Geometry: final body of the model. Coordinates: model frame, mm. A direction names the side the tool comes from. Round coordinates to 2 decimals unless told otherwise and drop trailing zeros. Loops run counter-clockwise (first coordinate to the right, second up) from the corner with the lowest first, then second, coordinate; pieces in that order, holes last. Notation, with made-up numbers: (8, -27) - (27, -27) arc R9 cw to (27, -13) - close; hole circle Ø4 at (-11.5, -23). An arc over 180 degrees is marked (long way). Answer as CSV lines item,"result".
from build123d import *

# Parameters (mm, degrees)
BOSS_EXTRUDE1_DEPTH       = 76.2
TAP_DRILL_FOR_6_32_TAP1_D = 2.7051


with BuildPart() as part:
    # Sketch2 → Boss-Extrude1 (new body)
    with BuildSketch(Plane.XY):
        with BuildLine():
            Line((-19.425899611, -6.35), (-6.35, -6.35))
            Line((-6.35, -6.35), (-6.35, 0))
            ThreePointArc((-6.35, 0), (0, 6.35), (6.35, 0))
            Line((6.35, 0), (6.35, -6.35))
            Line((6.35, -6.35), (19.425899611, -6.35))
            Line((19.425899611, -6.35), (19.425899611, -3.175))
            Line((19.425899611, -3.175), (12.7, -3.175))
            Line((12.7, -3.175), (12.7, 0))
            ThreePointArc((12.7, 0), (0, 12.7), (-12.7, 0))
            Line((-12.7, 0), (-12.7, -3.175))
            Line((-12.7, -3.175), (-19.425899611, -3.175))
            Line((-19.425899611, -3.175), (-19.425899611, -6.35))
        make_face()
    extrude(amount=BOSS_EXTRUDE1_DEPTH)

    # Tap Drill for #6-32 Tap1 (through all)
    with Locations(Plane(origin=(0, -3.175, 0), x_dir=(1, 0, 0), z_dir=(0, 1, 0))):
        with Locations((-16.062949805, -38.1), (16.062949805, -38.1)):
            Hole(TAP_DRILL_FOR_6_32_TAP1_D / 2)


solid = part.part
(1) Pin query (flat end, axial travel): P1, Ø2.5, axis at x = 16.06, z = 38.1, coming from the -Y side; P2, Ø5, axis at x = -1.5, z = 25, coming from the -Y side; P3, Ø3, axis at y = -1, z = 21.5, coming from the -X side; P4, Ø5, axis at x = -9.5, z = 36.5, coming from the +Y side. Return the tip coordinate at first contact, or that it passes through.
Findings below:
P1,"through"
P2,"y = 4.93"
P3,"x = -12.7"
P4,"y = 10.6"
(2) Section B-B (z = 50.5). Output: boundary loops of the cut face in (x, y) (3 decimals).
Findings below:
outline,"(-19.426, -6.35) - (-6.35, -6.35) - (-6.35, 0) arc R6.35 cw to (6.35, 0) - (6.35, -6.35) - (19.426, -6.35) - (19.426, -3.175) - (12.7, -3.175) - (12.7, 0) arc R12.7 ccw to (-12.7, 0) - (-12.7, -3.175) - (-19.426, -3.175) - close"
(3) Section C-C (x = 0). Output: boundary loops of the cut face in (y, z).
Findings below:
outline,"(6.35, 0) - (12.7, 0) - (12.7, 76.2) - (6.35, 76.2) - close"
(4) Section D-D (y = 8.5). Output: boundary loops of the cut face in (x, z), and give its area (3 significant figures).
Findings below:
outline,"(-9.44, 0) - (9.44, 0) - (9.44, 76.2) - (-9.44, 76.2) - close"
area,"1,440 mm2"
(5) Draft query along X for faces 1 (the face through (15.44, -4.78, 39.3)), 2 (the face through (0.279, 12.697, 37.567)), 3 (the face through (-6.35, -3, 38)), 4 (the face through (-19.426, -5, 38)). Return one class per face: pulls with the +X half, pulls with the -X half, needs draft (parallel to the pull), parting line crosses it, or undercut.
Findings below:
face 1,"undercut"
face 2,"parting line crosses it"
face 3,"undercut"
face 4,"pulls with the -X half"
(6) Section A-A (x = -16.5). Output: boundary loops of the cut face in (y, z) (3 decimals), and give its area (3 significant figures).
Findings below:
outline,"(-6.35, 0) - (-3.175, 0) - (-3.175, 36.82) - (-6.35, 36.82) - close; (-6.35, 39.38) - (-3.175, 39.38) - (-3.175, 76.2) - (-6.35, 76.2) - close"
area,"234 mm2"
(7) Material intervals for line 1 along X through (y, z) = (-3.95, 38.1); line 2 along X through (y, z) = (-5.25, 62); line 3 along X through (y, z) = (-1, 70.5), sorted ascending.
Findings below:
line 1,"-19.43 to -17.42, -14.71 to -6.35, 6.35 to 14.71, 17.42 to 19.43"
line 2,"-19.43 to -6.35, 6.35 to 19.43"
line 3,"-12.7 to -6.35, 6.35 to 12.7"
(8) Access query for faces 5 (the face through (-18, -3.175, 38)), 6 (the face through (-14.99, -4.785, 38.923)), 7 (the face through (12.7, -2, 38)), 8 (the face through (6.35, -3, 38)), 9 (the face through (13, -6.35, 38)). Directions: +Z, -Z, +X, -X, +Y, -Y. A direction counts if a zero-diameter tool reaches every point of the face in a straight line with its end or side. Return the directions, or none.
Findings below:
face 5,"+Z, -Z, -X, +Y"
face 6,"+Y, -Y"
face 7,"+Z, -Z, +X, +Y"
face 8,"+Z, -Z, -Y"
face 9,"+Z, -Z, +X, -X, -Y"
